```python
from build123d import *

# Parameters (mm, degrees)
SKETCH_1_W          = 100
SKETCH_1_H          = 100
EXTRUDE_1_DEPTH     = 20
SKETCH_2_R          = 30
CUT_EXTRUDE_1_DEPTH = 20


with BuildPart() as part:
    # 草图1 → 凸台-拉伸1 (new body)
    with BuildSketch(Plane.XY):
        Rectangle(SKETCH_1_W, SKETCH_1_H)
    extrude(amount=EXTRUDE_1_DEPTH)

    # 草图2 → 切除-拉伸1 (cut)
    with BuildSketch(Plane.XY.offset(20)):
        Circle(SKETCH_2_R)
    extrude(amount=-CUT_EXTRUDE_1_DEPTH, mode=Mode.SUBTRACT)

    # 草图3 → M6 六角圆柱头螺钉的柱形沉头孔1 (revolve, cut)
    with BuildSketch(Plane(origin=(-38.736943886, -34.103248867, 20), x_dir=(0, -1, 0), z_dir=(1, 0, 0))):
        Polygon((0, 0), (0, 20), (3.3, 20), (3.3, 6.815021515), (3.325, 6.8), (5.5, 6.8), (5.5, 0), align=None)
    revolve(axis=Axis((-38.736943886, -34.103248867, 26.35), (0, 0, -1)), mode=Mode.SUBTRACT)


solid = part.part
```
Work out the finished part from the listing and answer in its coordinate system (mm). A direction names the side the tool comes from. Round coordinates to 2 decimals unless told otherwise and drop trailing zeros. Write each loop counter-clockwise with the first axis right and the second up, starting at its lowest first coordinate (ties: lowest second). Pieces come first, ordered by that corner, then holes. Notation, with made-up numbers: (79.25, -2) -> (115.25, -2) arc R15 cw to (115.25, 17) -> close; hole circle Ø11 at (-5, 45). An arc over 180 degrees is marked (long way). Write each question's results on one line, items separated by ' | '.
Q1. A flat-ended cylindrical pin translates along its axis: P1, Ø3.5, axis at x = -38.5, y = -36.5, coming from the +Z side. Find the tip coordinate at first contact, or state that the pin passes through.
Data:
P1: z = 13.2
Q2. Section C-C, the plane z = 1.5 is taken. Write down the section's boundary in (x, y).
Data:
outline: (-50, -50) -> (50, -50) -> (50, 50) -> (-50, 50) -> close; hole circle Ø6.6 at (-38.74, -34.1); hole circle Ø60 at (0, 0)
Q3. Straight lines are drawn through the part: line 1 along Y through (x, z) = (-34, 14); line 2 along Y through (x, z) = (-37.5, 17.5); line 3 along X through (y, z) = (-36, 18.25). For each, find the intervals that lie inside material, in ascending order. Write a range as [from, to].
Data:
line 1: [-50, -36.9], [-31.31, 50] | line 2: [-50, -39.46], [-28.74, 50] | line 3: [-50, -43.9], [-33.57, 50]
Q4. Which of the six approach directions +Z, -Z, +X, -X, +Y, -Y give full straight-line access (tool end or side, diameter ignored) to faces 1 (the flat face through (-23, 23, 0)), 2 (the flat face through (-35, -34, 13.2))?
Data:
face 1: -Z, +X, -X, +Y, -Y | face 2: +Z
Q5. Section B-B, the plane x = 13 is taken. Write down the section's boundary in (y, z), then the cut area to 3 significant figures.
Data:
outline: (-50, 0) -> (-27.04, 0) -> (-27.04, 20) -> (-50, 20) -> close; (27.04, 0) -> (50, 0) -> (50, 20) -> (27.04, 20) -> close | area: 919 mm^2
Q6. Determine the mould class of faces 3 (the cylindrical face through (-38.882, -30.806, 6.685)), 4 (the flat face through (-1, 50, 10)), 5 (the flat face through (22, 23, 20)) for opening direction Y: released by +Y, released by -Y, zero draft, split by the parting line, or undercut.
Data:
face 3: undercut | face 4: released by +Y | face 5: zero draft
Q7. Section A-A, the plane y = 0 is taken. Write down the section's boundary in (x, z).
Data:
outline: (-50, 0) -> (-30, 0) -> (-30, 20) -> (-50, 20) -> close; (30, 0) -> (50, 0) -> (50, 20) -> (30, 20) -> close
